For this review, take the finished solid that the model builds, in its own axes (mm). A direction names the side the tool comes from. Give positions to 0.01 mm unless a question says otherwise; leave off trailing zeros. Loops run counter-clockwise (first coordinate to the right, second up) from the corner with the lowest first, then second, coordinate; pieces in that order, holes last. Notation, with made-up numbers: (22, -14) -> (59, -14) arc R9 ccw to (59, 1) -> close; hole circle Ø2 at (20.25, 69.25). An arc over 180 degrees is marked (long way). One line per question, with ' | ' between items. Start each with the question number.
(1) Draft analysis for pull direction Y (two halves, no side actions). For faces 4 (the flat face through (-1, 10, 2)), 5 (the cylindrical face through (0, 1, 3)), 6 (the flat face through (-1, 0, 2)), state which applies: +Y half, -Y half, draft (parallel to the pull), parting line (faces both ways), or undercut.
(2) Consider section A-A (x = 0). Write out the cut boundary in (y, z).
(3) Consider section C-C (x = -1.5). Write out the cut boundary in (y, z), and give its area (3 significant figures).
(4) Tool access review of faces 1 (the cylindrical face through (3, 1, 0)), 2 (the cylindrical face through (-4.39, 4.93, -0.98)), 3 (the cylindrical face through (0, 7, 3)): name each direction out of +Z, -Z, +X, -X, +Y, -Y from which nothing blocks a thin tool from reaching the whole face with its end or side.
(5) Consider section B-B (z = 0). Write out the cut boundary in (x, y), and give its area (3 significant figures).
(6) Consider section D-D (y = 8). Write out the cut boundary in (x, z).
(7) Wall thickness on probe 1 along X at (y, z) = (6.5, 0); probe 2 along Z at (x, y) = (1.25, 4.75); probe 3 along X at (y, z) = (4, 0.5): over which ranges is each line inside the solid? List them lowest first.
(8) Insertion check: P1, Ø4, axis at x = 0.5, z = 0.5, coming from the +Y side; P2, Ø3, axis at y = 2.5, z = -2.5, coming from the +X side; P3, Ø1.5, axis at x = 2.5, y = 1.5, coming from the +Z side. Each pin has a flat end and moves straight along its axis. Give the tip position at first contact, or say it passes through.
from build123d import *

# Parameters (mm, degrees)
SKETCH1_R           = 4.5
SKETCH1_R_2         = 2
BOSS_EXTRUDE1_DEPTH = 10
SKETCH2_R           = 1
CUT_EXTRUDE1_DEPTH  = 12.853269591


with BuildPart() as part:
    # Sketch1 → Boss-Extrude1 (new body)
    with BuildSketch(Plane(origin=(0, 0, 0), x_dir=(1, 0, 0), z_dir=(0, 1, 0))):
        with Locations(Location((0, 0, 0), (0, 0, 270))):
            Circle(SKETCH1_R)
        with Locations(Location((0, 0, 0), (0, 0, 270))):
            Circle(SKETCH1_R_2, mode=Mode.SUBTRACT)
    extrude(amount=BOSS_EXTRUDE1_DEPTH)

    # Sketch2 → Cut-Extrude1 (cut, through all)
    with BuildSketch(Plane.XY):
        with Locations(Location((0, 8, 0), (0, 0, 270.000000002))):
            Circle(SKETCH2_R)
        with Locations(Location((0, 2, 0), (0, 0, 270.000000002))):
            Circle(SKETCH2_R)
    cut_extrude1 = extrude(amount=CUT_EXTRUDE1_DEPTH, mode=Mode.SUBTRACT)

    # Mirror1: Cut-Extrude1 across plane
    add(cut_extrude1.mirror(Plane(origin=(0, 0, 0), x_dir=(0.7071067811865465, 0, 0.7071067811865486), z_dir=(-0.7071067811865488, 0, 0.7071067811865464))), mode=Mode.SUBTRACT)


solid = part.part
A:
1) face 4: +Y half | face 5: undercut | face 6: -Y half
2) outline: (0, -4.5) -> (10, -4.5) -> (10, -2) -> (0, -2) -> close; (0, 2) -> (1, 2) -> (1, 4.5) -> (0, 4.5) -> close; (3, 2) -> (7, 2) -> (7, 4.5) -> (3, 4.5) -> close; (9, 2) -> (10, 2) -> (10, 4.5) -> (9, 4.5) -> close
3) outline: (0, -4.24) -> (10, -4.24) -> (10, -1.32) -> (0, -1.32) -> close; (0, 1.32) -> (10, 1.32) -> (10, 4.24) -> (0, 4.24) -> close | area: 58.4 mm^2
4) face 1: +X | face 2: +Y, -Y | face 3: +Z
5) outline: (-4.5, 0) -> (-2, 0) -> (-2, 10) -> (-4.5, 10) -> close; (2, 0) -> (4.5, 0) -> (4.5, 1) -> (2, 1) -> close; (2, 3) -> (4.5, 3) -> (4.5, 7) -> (2, 7) -> close; (2, 9) -> (4.5, 9) -> (4.5, 10) -> (2, 10) -> close | area: 40.0 mm^2
6) outline: (-1, 1.73) -> (-1, 4.39) arc R4.5 ccw (long way) to (4.39, -1) -> (1.73, -1) arc R2 cw (long way) to start; (1, 1.73) arc R2 cw to (1.73, 1) -> (4.39, 1) arc R4.5 ccw to (1, 4.39) -> close
7) probe 1: x = -4.5 to -2, 2 to 4.5 | probe 2: z = -4.32 to -1.56, 1.56 to 4.32 | probe 3: x = -4.47 to -1.94, 1.94 to 4.47
8) P1: stops at y = 10 | P2: stops at x = 4.39 | P3: stops at z = 4.15
